Source: CAD feature listing. Evaluate the final solid. Frame: model axes, mm. Face numbers are marked on the shaded views. A direction names the side the tool comes from. Give positions to 0.01 mm unless a question says otherwise; leave off trailing zeros. Order: outer loops, then holes, each group sorted by start corner. A loop starts at its lowest first (then second) coordinate and runs counter-clockwise, first axis right, second up.
from build123d import *

# Parameters (mm, degrees)
BOSS_EXTRUDE1_DEPTH      = 22.606
BOSS_EXTRUDE1_DEPTH_BACK = 22.606
SKETCH1_5_W              = 6.35
SKETCH1_5_H              = 25.4
SKETCH1_5_H_2            = 9.906
BOSS_EXTRUDE2_DEPTH      = 22.86
BOSS_EXTRUDE3_DEPTH      = 6.35


with BuildPart() as part:
    # Sketch1 → Boss-Extrude1 (new, two sides: drawn at the far end of the back side and taken through both)
    with BuildSketch(Plane.YZ.offset(-BOSS_EXTRUDE1_DEPTH_BACK)):
        Polygon((6.35, 35.306), (6.35, 22.606), (62.23, 22.606), (62.23, 35.306), (62.23, 45.212), (6.35, 45.212), align=None)
        Polygon((0, 35.306), (0, 9.906), (6.35, 9.906), (6.35, 22.606), (6.35, 35.306), align=None)
        Polygon((6.35, 9.906), (6.35, 0), (62.23, 0), (62.23, 9.906), (62.23, 22.606), (6.35, 22.606), align=None)
        Polygon((62.23, 22.606), (62.23, 9.906), (68.58, 9.906), (68.58, 35.306), (62.23, 35.306), align=None)
    extrude(amount=BOSS_EXTRUDE1_DEPTH + BOSS_EXTRUDE1_DEPTH_BACK)

    # Sketch1_5 → Cut-Revolve3 (revolve, cut)
    with BuildSketch(Plane.YZ, mode=Mode.PRIVATE) as cut_revolve3_sk:
        with Locations((65.405, 57.912)):
            Rectangle(SKETCH1_5_W, SKETCH1_5_H)
        with Locations((65.405, 40.259)):
            Rectangle(SKETCH1_5_W, SKETCH1_5_H_2)
        with Locations((3.175, 57.912)):
            Rectangle(SKETCH1_5_W, SKETCH1_5_H)
        with Locations((3.175, 40.259)):
            Rectangle(SKETCH1_5_W, SKETCH1_5_H_2)
    revolve(cut_revolve3_sk.sketch.rotate(Axis((0, 6.35, 22.606), (0, 1, 0)), 180), axis=Axis((0, 6.35, 22.606), (0, 1, 0)), mode=Mode.SUBTRACT)

    # Sketch2 → Boss-Extrude2 (add)
    with BuildSketch(Plane.XY.offset(45.212)):
        with BuildLine():
            ThreePointArc((3.175, 34.29), (-2.24506403, 36.53506403), (0, 31.115))
            Line((0, 31.115), (0, 34.29))
            Line((0, 34.29), (3.175, 34.29))
        make_face()
        with BuildLine():
            Line((0, 34.29), (0, 31.115))
            ThreePointArc((0, 31.115), (2.24506403, 32.04493597), (3.175, 34.29))
            Line((3.175, 34.29), (0, 34.29))
        make_face()
    extrude(amount=BOSS_EXTRUDE2_DEPTH)

    # Sketch2_3 → Boss-Extrude3 (add)
    with BuildSketch(Plane.XY.offset(45.212)):
        with BuildLine():
            ThreePointArc((6.35, 34.29), (-4.490128061, 38.780128061), (0, 27.94))
            Line((0, 27.94), (0, 31.115))
            ThreePointArc((0, 31.115), (-2.24506403, 36.53506403), (3.175, 34.29))
            Line((3.175, 34.29), (6.35, 34.29))
        make_face()
        with BuildLine():
            Line((0, 31.115), (0, 27.94))
            ThreePointArc((0, 27.94), (4.490128061, 29.799871939), (6.35, 34.29))
            Line((6.35, 34.29), (3.175, 34.29))
            ThreePointArc((3.175, 34.29), (2.24506403, 32.04493597), (0, 31.115))
        make_face()
    extrude(amount=BOSS_EXTRUDE3_DEPTH)


solid = part.part
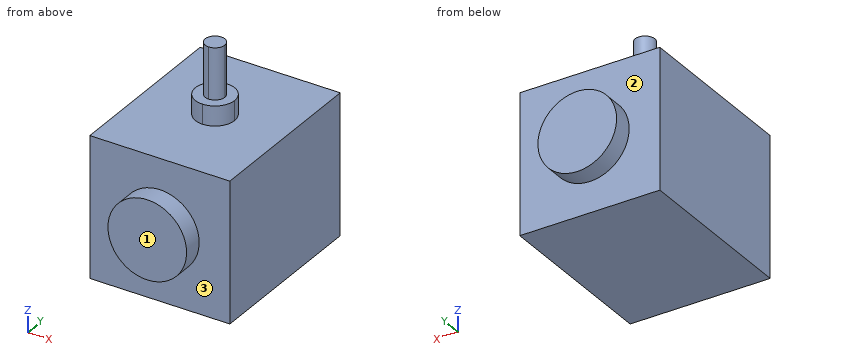
(1) Access query for the marked faces 1, 2 and 3. Directions: +Z, -Z, +X, -X, +Y, -Y. A direction counts if a zero-diameter tool reaches every point of the face in a straight line with its end or side. Return the directions, or none.
(2) Section A-A, the plane y = 32. Return loops of the section in (x, z).
(3) Section D-D, the plane x = -2. Return loops of the section in (y, z), plus the area to 3 significant figures.
(4) Section B-B, the plane x = 5. Return loops of the section in (y, z), plus the area to 3 significant figures.
(5) Line query: line 1 along Z through (x, y) = (13.5, 13); line 2 along Y through (x, z) = (-15.5, 4); line 3 along Y through (x, z) = (-4.5, 50.5). Output: solid intervals per line, ascending.
(6) Pin query (flat end, axial travel): pin 1 Ø12 at (x, y) = (-16, 58.5) entering from -Z; pin 2 Ø12 at (x, y) = (-2, 49) entering from +Z; pin 3 Ø5 at (x, z) = (-10.5, 38.5) entering from -Y. Return the tip coordinate at first contact, or that it passes through.
(7) Section C-C, the plane z = 22. Return loops of the section in (x, y).
Checks:
1. face 1: +Z, -Z, +X, -X, -Y
1. face 2: +Y
1. face 3: -Y
2. outline: (-22.61, 0) - (22.61, 0) - (22.61, 45.21) - (5.92, 45.21) - (5.92, 51.56) - (2.2, 51.56) - (2.2, 68.07) - (-2.2, 68.07) - (-2.2, 51.56) - (-5.92, 51.56) - (-5.92, 45.21) - (-22.61, 45.21) - close
3. outline: (0, 10.06) - (6.35, 10.06) - (6.35, 0) - (62.23, 0) - (62.23, 10.06) - (68.58, 10.06) - (68.58, 35.15) - (62.23, 35.15) - (62.23, 45.21) - (40.32, 45.21) - (40.32, 51.56) - (36.76, 51.56) - (36.76, 68.07) - (31.82, 68.07) - (31.82, 51.56) - (28.26, 51.56) - (28.26, 45.21) - (6.35, 45.21) - (6.35, 35.15) - (0, 35.15) - close
3. area: 3,000 mm2
4. outline: (0, 10.93) - (6.35, 10.93) - (6.35, 0) - (62.23, 0) - (62.23, 10.93) - (68.58, 10.93) - (68.58, 34.28) - (62.23, 34.28) - (62.23, 45.21) - (38.2, 45.21) - (38.2, 51.56) - (30.38, 51.56) - (30.38, 45.21) - (6.35, 45.21) - (6.35, 34.28) - (0, 34.28) - close
4. area: 2,870 mm2
5. line 1: z = 0 to 45.21
5. line 2: y = 6.35 to 62.23
5. line 3: y = 29.81 to 38.77
6. pin 1: stops at z = 0
6. pin 2: stops at z = 45.21
6. pin 3: stops at y = 6.35
7. outline: (-22.61, 6.35) - (-12.69, 6.35) - (-12.69, 0) - (12.69, 0) - (12.69, 6.35) - (22.61, 6.35) - (22.61, 62.23) - (12.69, 62.23) - (12.69, 68.58) - (-12.69, 68.58) - (-12.69, 62.23) - (-22.61, 62.23) - close
